from build123d import *

# Parameters (mm, degrees)
F0_W      = 25.4
F0_H      = 19.05
F1_DEPTH  = 19.05
F4_DEPTH  = 6.35
F5_R      = 4.445
F5_R_2    = 3.175
F6_DEPTH  = 6.35
F7_W      = 3.81
F7_H      = 1.27
F8_DEPTH  = 6.35
F10_DEPTH = 6.35
F11_W     = 1.905
F11_H     = 8.89
F12_DEPTH = 6.35
F14_DEPTH = 6.35
F15_W     = 1.27
F15_H     = 1.27
F16_DEPTH = 6.35
F18_DEPTH = 6.35
F19_W     = 3.81
F19_H     = 1.27
F20_DEPTH = 6.35


with BuildPart() as f1:
    # F0 (on Front) → F1 (new body)
    with BuildSketch(Plane.XZ):
        Polygon((-25.4, 0), (0, 0), (0, 57.15), (0, 76.2), (0, 101.6), (-25.4, 101.6), (-25.4, 76.2), (-25.4, 57.15), align=None)
        with Locations((12.7, 66.675)):
            Rectangle(F0_W, F0_H)
        with Locations((-38.1, 66.675)):
            Rectangle(F0_W, F0_H)
    extrude(amount=F1_DEPTH)

    # F3 (on offset) → F4 (join)
    with BuildSketch(Plane.XZ.offset(19.05)):
        Polygon((-45.72, 66.802), (-48.26, 66.802), (-48.26, 61.722), (-40.64, 61.722), (-40.64, 74.422), (-43.18, 74.422), (-43.18, 64.262), (-45.72, 64.262), align=None)
    extrude(amount=F4_DEPTH)

    # F5 (on offset) → F6 (join)
    with BuildSketch(Plane.XZ.offset(19.05)):
        with Locations((-33.655, 66.167)):
            Circle(F5_R)
        with Locations((-33.655, 66.167)):
            Circle(F5_R_2, mode=Mode.SUBTRACT)
    extrude(amount=F6_DEPTH)

    # F7 (on offset) → F8 (join)
    with BuildSketch(Plane.XZ.offset(19.05)):
        Polygon((-25.4, 70.612), (-26.67, 70.612), (-26.67, 61.722), (-25.4, 61.722), (-25.4, 65.786055), (-25.4, 67.056055), align=None)
        with Locations((-23.495, 66.421055)):
            Rectangle(F7_W, F7_H)
        Polygon((-21.59, 70.612), (-21.59, 67.056055), (-21.59, 65.786055), (-21.59, 61.722), (-20.32, 61.722), (-20.32, 70.612), align=None)
    extrude(amount=F8_DEPTH)

    # F9 (on offset) → F10 (join)
    with BuildSketch(Plane.XZ.offset(19.05)):
        Polygon((-17.78, 70.612), (-17.78, 61.722), (-16.51, 61.722), (-16.51, 68.510335), (-16.51, 70.612), align=None)
        Polygon((-12.917591, 63.891956), (-16.51, 70.612), (-16.51, 68.510335), (-13.048367, 61.722), (-12.917591, 61.722), align=None)
        Polygon((-12.917591, 70.612), (-12.917591, 63.891956), (-12.917591, 61.722), (-11.778367, 61.722), (-11.778367, 70.612), align=None)
    extrude(amount=F10_DEPTH)

    # F11 (on offset) → F12 (join)
    with BuildSketch(Plane.XZ.offset(19.05)):
        with Locations((-6.016459, 66.167)):
            Rectangle(F11_W, F11_H)
    extrude(amount=F12_DEPTH)

    # F13 (on offset) → F14 (join)
    with BuildSketch(Plane.XZ.offset(19.05)):
        Polygon((2.556041, 70.612), (-2.523959, 70.612), (-2.523959, 69.342), (0.651041, 69.342), (-2.523959, 62.344633), (-1.417059, 61.722), align=None)
    extrude(amount=F14_DEPTH)

    # F15 (on offset) → F16 (join)
    with BuildSketch(Plane.XZ.offset(19.05)):
        with Locations((5.731041, 67.945)):
            Rectangle(F15_W, F15_H)
        with Locations((5.731041, 64.135)):
            Rectangle(F15_W, F15_H)
    extrude(amount=F16_DEPTH)

    # F17 (on offset) → F18 (join)
    with BuildSketch(Plane.XZ.offset(19.05)):
        Polygon((13.986041, 70.612), (8.906041, 70.612), (8.906041, 69.342), (12.716041, 69.342), (12.716041, 66.802), (13.986041, 66.802), align=None)
        Polygon((13.986041, 65.532), (13.986041, 66.802), (12.716041, 66.802), (8.906041, 66.802), (8.906041, 61.722), (13.986041, 61.722), (13.986041, 62.992), (10.176041, 62.992), (10.176041, 65.532), align=None)
    extrude(amount=F18_DEPTH)

    # F19 (on offset) → F20 (join)
    with BuildSketch(Plane.XZ.offset(19.05)):
        with Locations((18.415, 69.977)):
            Rectangle(F19_W, F19_H)
        Polygon((20.32, 70.612), (20.32, 69.342), (20.32, 66.802), (20.32, 65.532), (20.32, 62.992), (20.32, 61.722), (21.59, 61.722), (21.59, 70.612), align=None)
        with Locations((18.415, 66.167)):
            Rectangle(F19_W, F19_H)
        with Locations((18.415, 62.357)):
            Rectangle(F19_W, F19_H)
    extrude(amount=F20_DEPTH)


solid = f1.part
Input: part model. Units: mm. Frame: model coordinates. A direction names the side the tool comes from. Give positions to 0.01 mm unless a question says otherwise; leave off trailing zeros. Order: outer loops, then holes, each group sorted by start corner. A loop starts at its lowest first (then second) coordinate and runs counter-clockwise, first axis right, second up. Notation, with made-up numbers: (39, -10.75) -> (59, -10.75) arc R4 ccw to (59, -3.75) -> close; hole circle Ø5 at (48, -9.75). An arc over 180 degrees is marked (long way). Use one line per item in the form item = value.
1) Section B-B, the plane y = -20.25. Count the separate pieces of the cut face and the enclosed holes in it, and give its area (3 significant figures).
Response values:
separate_pieces = 10
enclosed_holes = 1
area = 227 mm^2
2) Reachability of faces 1 (the flat face through (-43.18, -22, 69)), 2 (the flat face through (13.986, -22, 68)), 3 (the flat face through (-21.59, -22, 64)), 4 (the flat face through (11, -22, 66.802)) from +Z, -Z, +X, -X, +Y, -Y: full face, straight path, thin tool, end or side. Return the list, or none.
Response values:
face_1 = +Z, -Y
face_2 = +Z, -Z, -Y
face_3 = -Z, -Y
face_4 = -Y
3) Section A-A, the plane y = -4.5. Return loops of the section in (x, z).
Response values:
outline = (-50.8, 57.15) -> (-25.4, 57.15) -> (-25.4, 0) -> (0, 0) -> (0, 57.15) -> (25.4, 57.15) -> (25.4, 76.2) -> (0, 76.2) -> (0, 101.6) -> (-25.4, 101.6) -> (-25.4, 76.2) -> (-50.8, 76.2) -> close
4) Line query: probe 1 along Z at (x, y) = (19.5, -13.75); probe 2 along Y at (x, z) = (-37, 58); probe 3 along X at (y, z) = (-16.5, 80.5). Output: solid intervals per line, ascending.
Response values:
probe_1 = 57.15 to 76.2
probe_2 = -19.05 to 0
probe_3 = -25.4 to 0
5) Section C-C, the plane z = 27.5. Return loops of the section in (x, y), and give its area (3 significant figures).
Response values:
outline = (-25.4, -19.05) -> (0, -19.05) -> (0, 0) -> (-25.4, 0) -> close
area = 484 mm^2
6) Mould query, pull axis X, two halves, no side actions, for faces 5 (the flat face through (-43, -25.4, 67)), 6 (the flat face through (25.4, -9, 67)), 7 (the flat face through (18, -22, 62.992)). Classes: pulls with the +X half, pulls with the -X half, needs draft (parallel to the pull), parting line crosses it, or undercut.
Response values:
face_5 = needs draft
face_6 = pulls with the +X half
face_7 = undercut
7) First-contact query: pin 1 Ø9.5 at (y, z) = (-7, 31) entering from -X; pin 2 Ø4 at (x, y) = (17.5, -21) entering from +Z; pin 3 Ø2 at (y, z) = (-22.5, 64) entering from +X. Flat tips, straight axial feed; report the tip coordinate or a pass-through.
Response values:
pin_1 = -25.4
pin_2 = 76.2
pin_3 = 21.59
